Check sheet for the drawn part. Datum: minimum x, y, z corner. Units: mm. Coordinates: 2 decimals unless noted, no trailing zeros. Order: outer loops, then holes, each group sorted by start corner. A loop starts at its lowest first (then second) coordinate and runs counter-clockwise, first axis right, second up. Notation, with made-up numbers: (3.5, 86) - (8.5, 86) arc R21 cw to (8.5, 90) - close; hole circle Ø1 at (53.5, 45.25). An arc over 180 degrees is marked (long way). Return JSON: item names as keys, results as strings. Group by question number.
Item 1: Scan lines: probe 1 along Z at (x, y) = (10, 122.5); probe 2 along Z at (x, y) = (17, 250.5); probe 3 along Y at (x, z) = (1.25, 360). Record each from-to range of solid material in increasing order.
Item 2: Section check C-C on y = 39. Enter the section's corners in (x, z), then the cut area to 3 significant figures.
Item 3: Section check D-D on z = 794. Enter the section's corners in (x, y), then the cut area to 3 significant figures.
Item 4: Section check A-A on y = 142. Enter the section's corners in (x, z).
Item 5: Section check B-B on x = 6.75. Give the number of separate pieces and of enclosed holes in the cut face, then the cut area to 3 significant figures.
Item 6: Gauge pin test, flat ends, axial feed: pin 1 (1.5 mm diameter, centred on x = 5.5, y = 328.5, fed in from -Z); pin 2 (5.5 mm diameter, centred on x = 13, z = 369, fed in from -Y); pin 3 (4 mm diameter, centred on x = 2, z = 391, fed in from +Y); pin 4 (5.5 mm diameter, centred on x = 14, z = 900.5, fed in from +Y). Record the tip position at first contact, or that the pin passes through.
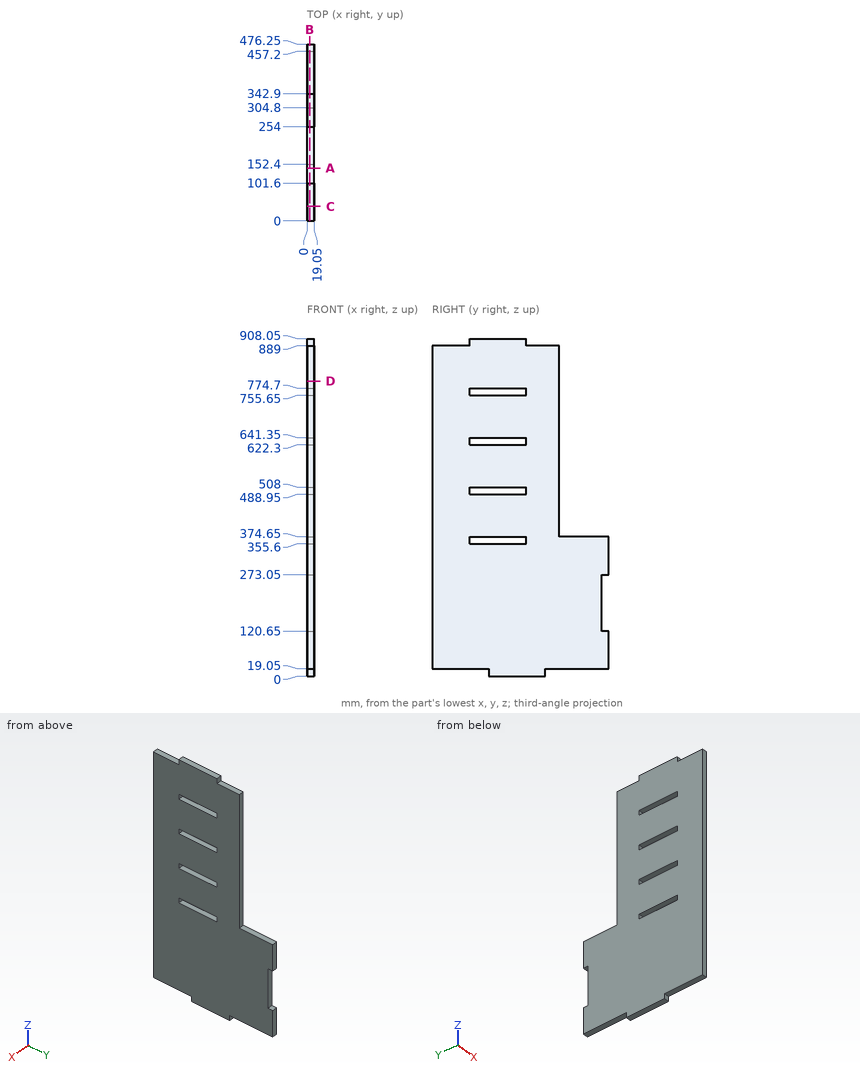
Computed:
{
 "1": {"probe 1": "z = 19.05 to 355.6, 374.65 to 488.95, 508 to 622.3, 641.35 to 755.65, 774.7 to 908.05", "probe 2": "z = 0 to 355.6, 374.65 to 488.95, 508 to 622.3, 641.35 to 755.65, 774.7 to 908.05", "probe 3": "y = 0 to 101.6, 254 to 476.25"},
 "2": {"outline": "(0, 19.05) - (19.05, 19.05) - (19.05, 889) - (0, 889) - close", "area": "16,600 mm²"},
 "3": {"outline": "(0, 0) - (19.05, 0) - (19.05, 342.9) - (0, 342.9) - close", "area": "6,530 mm²"},
 "4": {"outline": "(0, 19.05) - (19.05, 19.05) - (19.05, 355.6) - (0, 355.6) - close; (0, 374.65) - (19.05, 374.65) - (19.05, 488.95) - (0, 488.95) - close; (0, 508) - (19.05, 508) - (19.05, 622.3) - (0, 622.3) - close; (0, 641.35) - (19.05, 641.35) - (19.05, 755.65) - (0, 755.65) - close; (0, 774.7) - (19.05, 774.7) - (19.05, 908.05) - (0, 908.05) - close"},
 "5": {"separate pieces": "1", "enclosed holes": "4", "area": "337,000 mm²"},
 "6": {"pin 1": "stops at z = 19.05", "pin 2": "stops at y = 0", "pin 3": "stops at y = 342.9", "pin 4": "stops at y = 254"}
}
